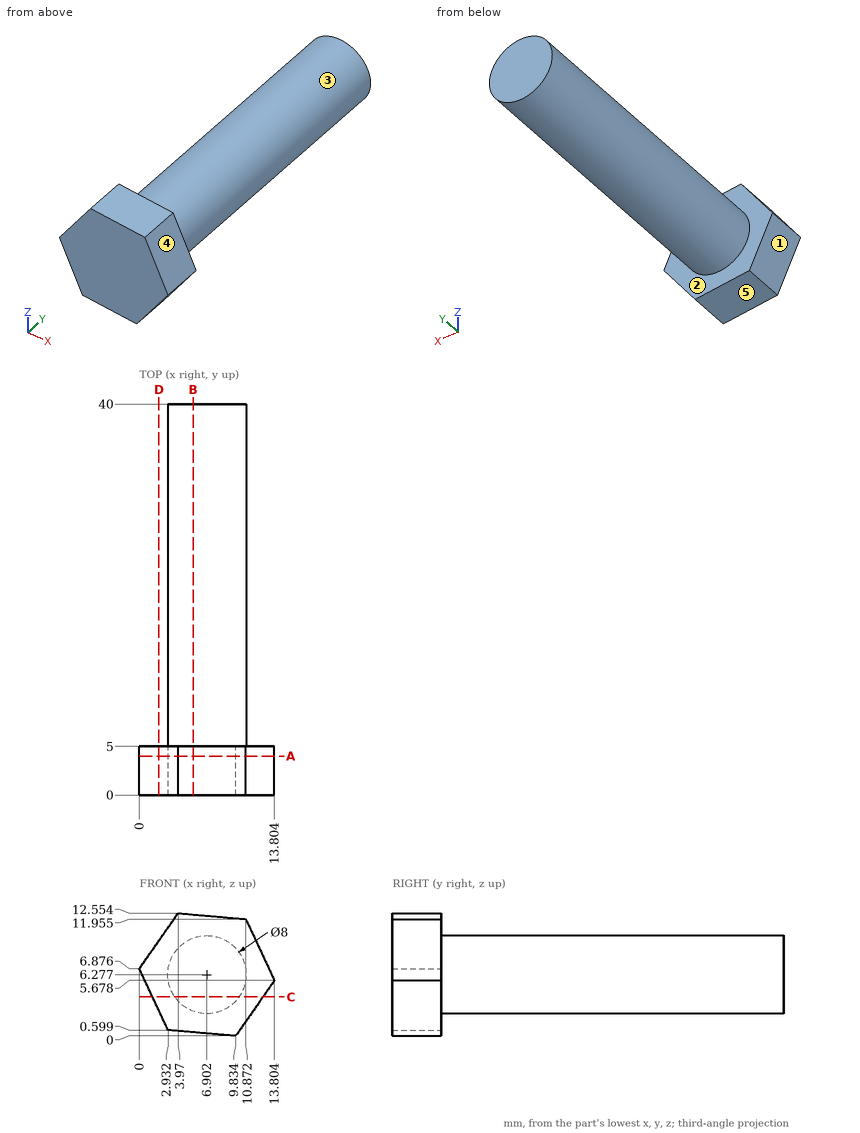
The drawing under review shows one solid part. Ordinate dimensions are in mm from its lowest x, y, z. A direction names the side the tool comes from. Give positions to 0.01 mm unless a question says otherwise; leave off trailing zeros. Write each loop counter-clockwise with the first axis right and the second up, starting at its lowest first coordinate (ties: lowest second). Pieces come first, ordered by that corner, then holes. Notation, with made-up numbers: (56.5, -17.5) - (102.5, -17.5) arc R21 cw to (102.5, 7.5) - close; hole circle Ø5 at (-9, 80.25). An arc over 180 degrees is marked (long way). Answer in a Markdown table with one row per item. Add a question column.
1. We need section C-C on z = 4. Write out the cut boundary in (x, y), then the cut area to 3 significant figures.
2. We need section A-A on y = 4. Write out the cut boundary in (x, z) (1 decimal).
3. Insertion check: P1, Ø1, axis at x = 4.5, y = 14.5, coming from the +Z side (1 decimal); P2, Ø2, axis at y = 7, z = 5.5, coming from the -X side; P3, Ø2, axis at x = 2, z = 9, coming from the +Y side. Each pin has a flat end and moves straight along its axis. Give the tip position at first contact, or say it passes through.
4. We need section D-D on x = 2. Write out the cut boundary in (y, z) (1 decimal), then the cut area to 3 significant figures.
5. Tool access review of the marked faces 1 and 2: name each direction out of +Z, -Z, +X, -X, +Y, -Y from which nothing blocks a thin tool from reaching the whole face with its end or side.
6. Wall thickness on line 1 along X through (y, z) = (15, 6.5) (1 decimal); line 2 along Y through (x, z) = (6.75, 12.25); line 3 along Z through (x, y) = (8.5, 11) (1 decimal): over which ranges is each line inside the solid? List them lowest first. Write a range as [from, to].
7. We need section B-B on x = 5.5. Write out the cut boundary in (y, z).
8. Draft analysis for pull direction X (two halves, no side actions). For the marked faces 3, 4 and 5, state which applies: +X half, -X half, draft (parallel to the pull), parting line (faces both ways), or undercut.
Ans:
| question | item | result |
|---|---|---|
| 1 | outline | (1.34, 0) - (12.63, 0) - (12.63, 5) - (10.19, 5) - (10.19, 40) - (3.61, 40) - (3.61, 5) - (1.34, 5) - close |
| 1 | area | 287 mm^2 |
| 2 | outline | (0, 6.9) - (2.9, 0.6) - (9.8, 0) - (13.8, 5.7) - (10.9, 12) - (4, 12.6) - close |
| 3 | P1 | stops at z = 9.8 |
| 3 | P2 | stops at x = 2.9 |
| 3 | P3 | stops at y = 5 |
| 4 | outline | (0, 2.6) - (5, 2.6) - (5, 9.7) - (0, 9.7) - close |
| 4 | area | 35.7 mm^2 |
| 5 | face 1 | -Z, -X, +Y, -Y |
| 5 | face 2 | +Y |
| 6 | line 1 | x = [2.9, 10.9] |
| 6 | line 2 | y = [0, 5] |
| 6 | line 3 | z = [2.6, 9.9] |
| 7 | outline | (0, 0.38) - (5, 0.38) - (5, 2.53) - (40, 2.53) - (40, 10.02) - (5, 10.02) - (5, 12.42) - (0, 12.42) - close |
| 8 | face 3 | parting line |
| 8 | face 4 | +X half |
| 8 | face 5 | -X half |
